Verification items for the finished model (mm, model axes). A direction names the side the tool comes from. Round coordinates to 2 decimals unless told otherwise and drop trailing zeros. Order: outer loops, then holes, each group sorted by start corner. A loop starts at its lowest first (then second) coordinate and runs counter-clockwise, first axis right, second up. Notation, with made-up numbers: (26, 53) -> (63, 53) arc R37 ccw to (63, 92) -> close; hole circle Ø9 at (47, -26). An arc over 180 degrees is marked (long way). Put each result on its own line as item: value.
```python
from build123d import *

# Parameters (mm, degrees)
SKETCH1_W           = 28
SKETCH1_H           = 28
BOSS_EXTRUDE1_DEPTH = 46
SKETCH2_W           = 28
SKETCH2_H           = 28
SKETCH2_R           = 11
CUT_EXTRUDE1_DEPTH  = 15
SKETCH3_R           = 2.5
BOSS_EXTRUDE2_DEPTH = 20


with BuildPart() as part:
    # Sketch1 → Boss-Extrude1 (new body)
    with BuildSketch(Plane.XY):
        with Locations((14, -14)):
            Rectangle(SKETCH1_W, SKETCH1_H)
    extrude(amount=BOSS_EXTRUDE1_DEPTH)

    # Sketch2 → Cut-Extrude1 (cut)
    with BuildSketch(Plane.XY.offset(46)):
        with Locations((14, -14)):
            Rectangle(SKETCH2_W, SKETCH2_H)
        with Locations((14, -14)):
            Circle(SKETCH2_R, mode=Mode.SUBTRACT)
    extrude(amount=-CUT_EXTRUDE1_DEPTH, mode=Mode.SUBTRACT)

    # Sketch3 → Boss-Extrude2 (add)
    with BuildSketch(Plane(origin=(0, 0, 0), x_dir=(-1, 0, 0), z_dir=(0, 0, -1))):
        with Locations((-14, -14)):
            Circle(SKETCH3_R)
    extrude(amount=BOSS_EXTRUDE2_DEPTH)


solid = part.part
```
Item 1: Material ranges on line 1 along Z through (x, y) = (22.5, -26); line 2 along Z through (x, y) = (23.5, -15.75); line 3 along X through (y, z) = (-13.75, 39.5), recorded low to high.
Geometry check:
line 1: 0 to 31
line 2: 0 to 46
line 3: 3 to 25
Item 2: Sectioned sample at A-A, the plane x = 14. Record the boundary of the cut face in (y, z), then the cut area to 3 significant figures.
Geometry check:
outline: (-28, 0) -> (-16.5, 0) -> (-16.5, -20) -> (-11.5, -20) -> (-11.5, 0) -> (0, 0) -> (0, 31) -> (-3, 31) -> (-3, 46) -> (-25, 46) -> (-25, 31) -> (-28, 31) -> close
area: 1,300 mm2
Item 3: Sectioned sample at B-B, the plane y = -14. Record the boundary of the cut face in (x, z).
Geometry check:
outline: (0, 0) -> (11.5, 0) -> (11.5, -20) -> (16.5, -20) -> (16.5, 0) -> (28, 0) -> (28, 31) -> (25, 31) -> (25, 46) -> (3, 46) -> (3, 31) -> (0, 31) -> close
Item 4: Depth check by flat-ended pin: pin 1 Ø2 at (x, z) = (14.5, -4) entering from +Y; pin 2 Ø1.5 at (y, z) = (-18, 6.5) entering from -X; pin 3 Ø3 at (x, y) = (23, -24) entering from -Z. Enter the tip coordinate at first touch or a pass-through.
Geometry check:
pin 1: y = -11.5
pin 2: x = 0
pin 3: z = 0
Item 5: Sectioned sample at C-C, the plane z = 32. Record the boundary of the cut face in (x, y).
Geometry check:
outline: circle Ø22 at (14, -14)
Item 6: Sectioned sample at D-D, the plane x = 24.25. Record the boundary of the cut face in (y, z), then the cut area to 3 significant figures.
Geometry check:
outline: (-28, 0) -> (0, 0) -> (0, 31) -> (-10.01, 31) -> (-10.01, 46) -> (-17.99, 46) -> (-17.99, 31) -> (-28, 31) -> close
area: 988 mm2
Item 7: Tool access check on faces 1 (the face through (28, -14, 15)), 2 (the face through (11.62, -24.74, 38.61)), 3 (the face through (16, -15.5, -9.9)). Record the directions out of +Z, -Z, +X, -X, +Y, -Y that give a thin tool (end or side, any length) a straight path to the whole face; none if there is none.
Geometry check:
face 1: +Z, -Z, +X, +Y, -Y
face 2: +Z
face 3: -Z
